For this review, use the dimensioned drawing (mm, ordinates from the lowest corner) and the shaded views. Round coordinates to 2 decimals unless told otherwise and drop trailing zeros. Write each loop counter-clockwise with the first axis right and the second up, starting at its lowest first coordinate (ties: lowest second). Pieces come first, ordered by that corner, then holes.
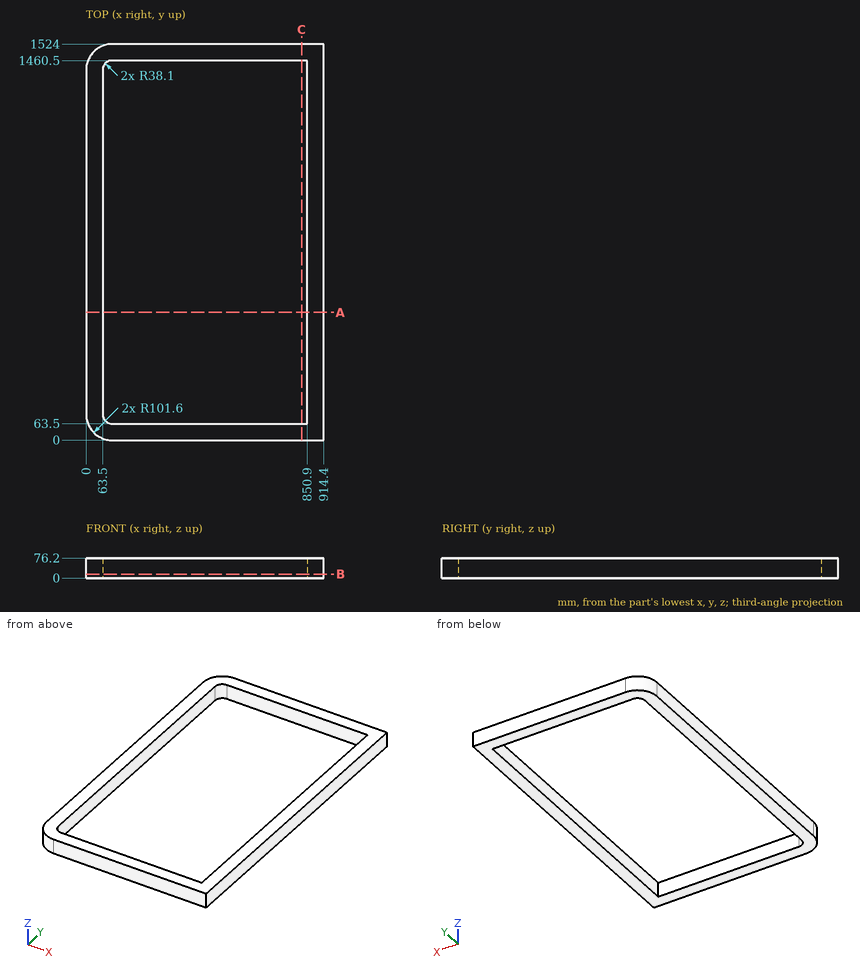
(1) We need section B-B, the plane z = 15. Give the boundary of the cut face in (x, y).
Geometry check:
outline: (0, 101.6) arc R101.6 ccw to (101.6, 0) - (914.4, 0) - (914.4, 1524) - (101.6, 1524) arc R101.6 ccw to (0, 1422.4) - close; hole (63.5, 101.6) arc R38.1 ccw to (101.6, 63.5) - (850.9, 63.5) - (850.9, 1460.5) - (101.6, 1460.5) arc R38.1 ccw to (63.5, 1422.4) - close
(2) We need section C-C, the plane x = 829. Give the boundary of the cut face in (y, z).
Geometry check:
outline: (0, 0) - (63.5, 0) - (63.5, 76.2) - (0, 76.2) - close; (1460.5, 0) - (1524, 0) - (1524, 76.2) - (1460.5, 76.2) - close
(3) We need section A-A, the plane y = 491.5. Give the boundary of the cut face in (x, z), and give its area (3 significant figures).
Geometry check:
outline: (0, 0) - (63.5, 0) - (63.5, 76.2) - (0, 76.2) - close; (850.9, 0) - (914.4, 0) - (914.4, 76.2) - (850.9, 76.2) - close
area: 9,680 mm2
(4) For line 1 along X through (y, z) = (456.5, 9); line 2 along Y through (x, z) = (747, 4.5); line 3 along X through (y, z) = (84, 46), list the stretches that pass through material, from the lowest coordinate up.
Geometry check:
line 1: x = 0 to 63.5, 850.9 to 914.4
line 2: y = 0 to 63.5, 1460.5 to 1524
line 3: x = 1.54 to 67.81, 850.9 to 914.4
